Design review of the part built by this model. Coordinates are the model's own, in mm. Round coordinates to 2 decimals unless told otherwise and drop trailing zeros. Loops run counter-clockwise (first coordinate to the right, second up) from the corner with the lowest first, then second, coordinate; pieces in that order, holes last. Notation, with made-up numbers: (77.5, 87) -> (127.5, 87) arc R19 cw to (127.5, 123) -> close; hole circle Ø3 at (15.25, 56). An arc over 180 degrees is marked (long way). Use a Markdown table: item, result. Add a question column.
from build123d import *

# Parameters (mm, degrees)
SKETCH1_R          = 2.413
EXTRUDE1_DEPTH     = 4.4958
CUT_EXTRUDE1_DEPTH = 114.681186736
FILLET1_R          = 6.35


with BuildPart() as part:
    # Sketch1 → Extrude1 (new body)
    with BuildSketch(Plane.XY):
        Polygon((26.2420825, 50.8), (0, 23.368), (0, 0), (101.6, 0), (101.6, 23.368), (70.6920825, 38.090460221), (38.9420825, 50.8), align=None)
        with Locations((20.32, 31.75)):
            Circle(SKETCH1_R, mode=Mode.SUBTRACT)
        with Locations((50.8, 9.525)):
            Circle(SKETCH1_R, mode=Mode.SUBTRACT)
        with Locations((85.09, 22.225)):
            Circle(SKETCH1_R, mode=Mode.SUBTRACT)
    extrude(amount=EXTRUDE1_DEPTH)

    # Sketch2 → Cut-Extrude1 (cut, through all)
    with BuildSketch(Plane.XY.offset(4.4958)):
        with BuildLine():
            Line((18.740269579, 42.958025871), (0, 23.368))
            Line((0, 23.368), (0, 0))
            Line((0, 0), (37.094444241, 0))
            ThreePointArc((37.094444241, 0), (13.737070061, 15.420367169), (18.740269579, 42.958025871))
        make_face()
        with BuildLine():
            Line((101.6, 23.368), (101.6, 0))
            Line((101.6, 0), (70.976404914, 0))
            ThreePointArc((70.976404914, 0), (90.236908542, 6.509249219), (101.6, 23.368))
        make_face()
    extrude(amount=-CUT_EXTRUDE1_DEPTH, mode=Mode.SUBTRACT)

    # Fillet1
    # the kernel refuses this fillet: 6.35 mm, written as the material it takes off along each edge
    with BuildSketch(Plane(origin=(26.2420825, 50.8, -6.782726088), x_dir=(-0.6912608610672895, -0.7226053016388058, 0), z_dir=(0, 0, 1))) as fillet1_piece_1:
        with BuildLine():
            CenterArc((FILLET1_R * 0.427258336235, FILLET1_R), FILLET1_R, 223.73, 46.27)
            Line((-FILLET1_R * 0.295346965404, FILLET1_R * 0.308739138933), (0, 0))
            Line((0, 0), (FILLET1_R * 0.427258336235, 0))
        make_face()
    extrude(amount=18.061252175, mode=Mode.SUBTRACT)
    with BuildSketch(Plane(origin=(38.9420825, 50.8, -3.059377728), x_dir=(-1, 0, 0), z_dir=(0, 0, 1))) as fillet1_piece_2:
        with BuildLine():
            CenterArc((FILLET1_R * 0.192716707281, FILLET1_R), FILLET1_R, 248.183751186, 21.816248814)
            Line((-FILLET1_R * 0.178914427547, FILLET1_R * 0.0716195286272), (0, 0))
            Line((0, 0), (FILLET1_R * 0.192716707281, 0))
        make_face()
    extrude(amount=10.614555456, mode=Mode.SUBTRACT)
    with BuildSketch(Plane(origin=(70.6920825, 38.090460221, -0.506345886), x_dir=(-0.9283804713727851, 0.3716311348281322, 0), z_dir=(0, 0, 1))) as fillet1_piece_3:
        with BuildLine():
            CenterArc((FILLET1_R * 0.0318958038441, FILLET1_R), FILLET1_R, 266.346248814, 3.653751186)
            Line((-FILLET1_R * 0.0318309718993, FILLET1_R * 0.00203261673873), (0, 0))
            Line((0, 0), (FILLET1_R * 0.0318958038441, 0))
        make_face()
    extrude(amount=5.508491772, mode=Mode.SUBTRACT)
    with BuildSketch(Plane(origin=(101.6, 23.368, -16.387317761), x_dir=(-0.9028105756982961, 0.43003844526659585, 0), z_dir=(0, 0, 1))) as fillet1_piece_4:
        with BuildLine():
            CenterArc((5.862905037, 6.35), FILLET1_R, 178.312383947, 91.687616053)
            ThreePointArc((-0.484340643, 6.537008757), (-0.411321416, 3.25597162), (0, 0))
            Line((0, 0), (5.862905037, 0))
        make_face()
    extrude(amount=37.270435521, mode=Mode.SUBTRACT)


solid = part.part
1. Insertion check: P1, Ø1.5, axis at y = 8, z = 2, coming from the -X side; P2, Ø1.5, axis at y = 15.5, z = 1.5, coming from the +X side. Each pin has a flat end and moves straight along its axis. Give the tip position at first contact, or say it passes through.
2. Consider section C-C on z = 1.6. Give the number of separate pieces and of enclosed holes in the cut face, plus the area to 3 significant figures.
3. To check wall thickness, follow probe 1 along Y at (x, z) = (85.09, 1); probe 2 along Y at (x, z) = (50.8, 3.4); probe 3 along X at (y, z) = (3, 0.3). State the ranges of each line that lie inside material, in increasing order. Write a range as from..to.
4. Consider section B-B on y = 31.75. State the section outline as (x, z) points.
5. Mouldability with a two-part tool opening along X and no side actions: class faces 1 (the face through (48.39, 9.63, 2.22)), 2 (the face through (87.32, 4.53, 2.28)), 3 (the face through (19.797, 29.394, 2.216)), 4 (the face through (33, 50.8, 2)) as +X half, -X half, draft (parallel to the pull), parting line (faces both ways), or undercut.
6. Consider section D-D on x = 62. State the section outline as (y, z) points, plus the area to 3 significant figures.
7. Consider section A-A on x = 86.5. State the section outline as (y, z) points, plus the area to 3 significant figures.
Verdict:
| question | item | result |
|---|---|---|
| 1 | P1 | stops at x = 17.91 |
| 1 | P2 | stops at x = 98.69 |
| 2 | separate pieces | 1 |
| 2 | enclosed holes | 3 |
| 2 | area | 3,230 mm² |
| 3 | probe 1 | y = 3.31..19.81, 24.64..31.23 |
| 3 | probe 2 | y = 0..7.11, 11.94..46.05 |
| 3 | probe 3 | x = 25.12..84.45 |
| 4 | outline | (12.5, 0) -> (17.91, 0) -> (17.91, 4.5) -> (12.5, 4.5) -> close; (22.73, 0) -> (84, 0) -> (84, 4.5) -> (22.73, 4.5) -> close |
| 5 | face 1 | undercut |
| 5 | face 2 | +X half |
| 5 | face 3 | undercut |
| 5 | face 4 | draft |
| 6 | outline | (0, 0) -> (41.57, 0) -> (41.57, 4.5) -> (0, 4.5) -> close |
| 6 | area | 187 mm² |
| 7 | outline | (4.05, 0) -> (20.27, 0) -> (20.27, 4.5) -> (4.05, 4.5) -> close; (24.18, 0) -> (30.56, 0) -> (30.56, 4.5) -> (24.18, 4.5) -> close |
| 7 | area | 102 mm² |
